from build123d import *

# Parameters (mm, degrees)
BOSS_EXTRUDE2_DEPTH = 13
SKETCH2_R           = 5
BOSS_EXTRUDE3_DEPTH = 21
SKETCH4_R           = 2.5
CUT_EXTRUDE1_DEPTH  = 21


with BuildPart() as part:
    # Sketch1 → Boss-Extrude2 (new body)
    with BuildSketch(Plane.XY):
        with BuildLine():
            Line((-4.358898944, 9), (4.358898944, 9))
            ThreePointArc((4.358898944, 9), (7.071067812, 7.071067812), (9, 4.358898944))
            Line((9, 4.358898944), (9, -4.358898944))
            ThreePointArc((9, -4.358898944), (7.071067812, -7.071067812), (4.358898944, -9))
            Line((4.358898944, -9), (-4.358898944, -9))
            ThreePointArc((-4.358898944, -9), (-7.071067812, -7.071067812), (-9, -4.358898944))
            Line((-9, -4.358898944), (-9, 4.358898944))
            ThreePointArc((-9, 4.358898944), (-7.071067812, 7.071067812), (-4.358898944, 9))
        make_face()
    extrude(amount=BOSS_EXTRUDE2_DEPTH)

    # Sketch2 → Boss-Extrude3 (add)
    with BuildSketch(Plane.XY):
        with Locations(Location((0, 0, 0), (0, 0, 180))):
            Circle(SKETCH2_R)
    extrude(amount=BOSS_EXTRUDE3_DEPTH)

    # Sketch4 → Cut-Extrude1 (cut)
    with BuildSketch(Plane.XY):
        with Locations(Location((0, 0, 0), (0, 0, 180))):
            Circle(SKETCH4_R)
    extrude(amount=CUT_EXTRUDE1_DEPTH, mode=Mode.SUBTRACT)


solid = part.part
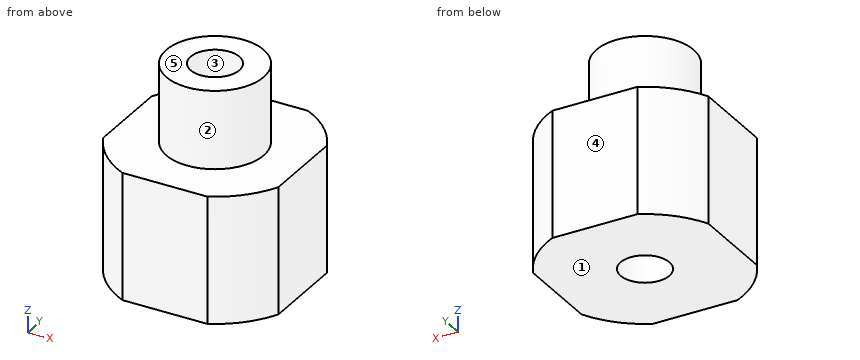
Model file for the job. Use its own axes, mm. Face numbers are marked on the shaded views. A direction names the side the tool comes from. Give positions to 0.01 mm unless a question says otherwise; leave off trailing zeros. Write each loop counter-clockwise with the first axis right and the second up, starting at its lowest first coordinate (ties: lowest second). Pieces come first, ordered by that corner, then holes. Notation, with made-up numbers: M 25,-10.5 L 58,-10.5 A22 cw 58,14.5 Z; hole C 73.25,54 d6. An arc over 180 degrees is marked long. One line per item, written item: value. Start each with the question number.
Q1. Probe probe 1 along Y at (x, z) = (0, 16.75); probe 2 along Y at (x, z) = (0, 9); probe 3 along Z at (x, y) = (-4, 6.25). List the from-to ranges inside material, lowest first. Write a range as [from, to].
Q2. Drop flat-ended pins along their axis: pin 1 Ø3 at (x, y) = (0, 6.5) entering from -Z; pin 2 Ø8 at (x, z) = (-6, 18) entering from +Y; pin 3 Ø3 at (x, z) = (1.5, 17.5) entering from +Y. Give the stop position or say it passes through.
Q3. Saw through at D-D, the plane y = 4. Write the cut outline in (x, z), plus the area to 3 significant figures.
Q4. Saw through at C-C, the plane z = 8.25. Write the cut outline in (x, y).
Q5. Saw through at A-A, the plane y = 0. Write the cut outline in (x, z), plus the area to 3 significant figures.
Q6. Two-plate mould, pull along Y, no slides. Class the marked faces 3, 4 and 5: +Y half, -Y half, draft (parallel to the pull), parting line (faces both ways), or undercut.
Q7. 3-axis set-ups, long thin cutter, end or side, ignore diameter. For the marked faces 1 and 2: which of +Z, -Z, +X, -X, +Y, -Y reach the whole face in a straight line?
Output values:
1. probe 1: y = [-5, -2.5], [2.5, 5]
1. probe 2: y = [-9, -2.5], [2.5, 9]
1. probe 3: z = [0, 13]
2. pin 1: stops at z = 0
2. pin 2: stops at y = 4.58
2. pin 3: stops at y = 5
3. outline: M -9,0 L 9,0 L 9,13 L 3,13 L 3,21 L -3,21 L -3,13 L -9,13 Z
3. area: 282 mm²
4. outline: M -9,-4.36 A10 ccw -4.36,-9 L 4.36,-9 A10 ccw 9,-4.36 L 9,4.36 A10 ccw 4.36,9 L -4.36,9 A10 ccw -9,4.36 Z; hole C 0,0 d5
5. outline: M -9,0 L -2.5,0 L -2.5,21 L -5,21 L -5,13 L -9,13 Z; M 2.5,0 L 9,0 L 9,13 L 5,13 L 5,21 L 2.5,21 Z
5. area: 209 mm²
6. face 3: undercut
6. face 4: +Y half
6. face 5: draft
7. face 1: -Z, +X, -X, +Y, -Y
7. face 2: +Z
